from build123d import *

# Parameters (mm, degrees)
SKETCH_1_R          = 60
EXTRUDE_1_DEPTH     = 8
SKETCH_3_R          = 9
EXTRUDE_3_DEPTH     = 36
SKETCH_4_R          = 60
EXTRUDE_4_DEPTH     = 8
SKETCH_5_R          = 15
EXTRUDE_5_DEPTH     = 48
SKETCH_6_R          = 3.3
CUT_EXTRUDE_1_DEPTH = 114.912246927
SKETCH_7_R          = 6
CUT_EXTRUDE_2_DEPTH = 114.912246927
SKETCH_8_R          = 20
CUT_EXTRUDE_3_DEPTH = 8
SKETCH_9_R          = 4.25
CUT_EXTRUDE_4_DEPTH = 20
CHAMFER_1_SIZE      = 1


with BuildPart() as part:
    # 草图1 → 凸台-拉伸1 (new body)
    with BuildSketch(Plane(origin=(0, 40, 0), x_dir=(1, 0, 0), z_dir=(0, 1, 0))):
        with Locations(Location((0, 0, 0), (0, 0, 270))):
            Circle(SKETCH_1_R)
    extrude(amount=EXTRUDE_1_DEPTH)

    # 草图3 → 凸台-拉伸3 (add)
    with BuildSketch(Plane(origin=(0, 40, 0), x_dir=(1, 0, 0), z_dir=(0, 1, 0))):
        with Locations(Location((45, 0, 0), (0, 0, 270))):
            Circle(SKETCH_3_R)
        with Locations(Location((-22.5, -38.971143, 0), (0, 0, 270))):
            Circle(SKETCH_3_R)
        with Locations(Location((-22.5, 38.971143, 0), (0, 0, 270))):
            Circle(SKETCH_3_R)
    extrude(amount=EXTRUDE_3_DEPTH)

    # 草图4 → 凸台-拉伸4 (add)
    with BuildSketch(Plane(origin=(0, 68, 0), x_dir=(1, 0, 0), z_dir=(0, 1, 0))):
        with Locations(Location((0, 0, 0), (0, 0, 270))):
            Circle(SKETCH_4_R)
    extrude(amount=EXTRUDE_4_DEPTH)

    # 草图5 → 凸台-拉伸5 (add)
    with BuildSketch(Plane(origin=(0, 0, 0), x_dir=(1, 0, 0), z_dir=(0, 1, 0))):
        with Locations(Location((0, 0, 0), (0, 0, 270))):
            Circle(SKETCH_5_R)
    extrude(amount=EXTRUDE_5_DEPTH)

    # 草图6 → 切除-拉伸1 (cut, through all)
    with BuildSketch(Plane(origin=(0, 76, 0), x_dir=(1, 0, 0), z_dir=(0, 1, 0))):
        with Locations(Location((45, 0, 0), (0, 0, 270))):
            Circle(SKETCH_6_R)
        with Locations(Location((-22.5, -38.971143, 0), (0, 0, 270))):
            Circle(SKETCH_6_R)
        with Locations(Location((-22.5, 38.971143, 0), (0, 0, 270))):
            Circle(SKETCH_6_R)
    extrude(amount=-CUT_EXTRUDE_1_DEPTH, mode=Mode.SUBTRACT)

    # 草图7 → 切除-拉伸2 (cut, through all)
    with BuildSketch(Plane(origin=(0, 76, 0), x_dir=(1, 0, 0), z_dir=(0, 1, 0))):
        with Locations(Location((22.5, -38.971143, 0), (0, 0, 270))):
            Circle(SKETCH_7_R)
        with Locations(Location((-45, 0, 0), (0, 0, 270))):
            Circle(SKETCH_7_R)
        with Locations(Location((22.5, 38.971143, 0), (0, 0, 270))):
            Circle(SKETCH_7_R)
    extrude(amount=-CUT_EXTRUDE_2_DEPTH, mode=Mode.SUBTRACT)

    # 草图8 → 切除-拉伸3 (cut)
    with BuildSketch(Plane(origin=(0, 76, 0), x_dir=(1, 0, 0), z_dir=(0, 1, 0))):
        with Locations(Location((0, 0, 0), (0, 0, 270))):
            Circle(SKETCH_8_R)
    extrude(amount=-CUT_EXTRUDE_3_DEPTH, mode=Mode.SUBTRACT)

    # 草图9 → 切除-拉伸4 (cut)
    with BuildSketch(Plane(origin=(0, 0, 0), x_dir=(1, 0, 0), z_dir=(0, 1, 0))):
        with Locations(Location((0, 0, 0), (0, 0, 270))):
            Circle(SKETCH_9_R)
    extrude(amount=CUT_EXTRUDE_4_DEPTH, mode=Mode.SUBTRACT)

    # 倒角1
    chamfer_1_edges = [part.edges().sort_by_distance(p)[0] for p in [
        (0, 40, -60),
        (0, 68, -60),
        (0, 76, -60),
        (0, 48, -60),
    ]]
    chamfer(chamfer_1_edges, length=CHAMFER_1_SIZE)


solid = part.part
For this review, take the finished solid that the model builds, in its own axes (mm). A direction names the side the tool comes from. Coordinates: 2 decimals unless noted, no trailing zeros. Loops run counter-clockwise (first coordinate to the right, second up) from the corner with the lowest first, then second, coordinate; pieces in that order, holes last. Notation, with made-up numbers: (-17.75, -20) - (13.25, -20) arc R9 cw to (13.25, -11) - close; hole circle Ø5 at (-39.5, -7). An arc over 180 degrees is marked (long way). Use a Markdown table: item, result. Add a question column.
Item 1: Mouldability with a two-part tool opening along Y and no side actions: class faces 5 (the face through (2.64, 71.96, -59.94)), 6 (the face through (-19.797, 57.86, -30.387)), 7 (the face through (-3.12, 0, 3.12)), 8 (the face through (1, 76, 25)) as pulls with the +Y half, pulls with the -Y half, needs draft (parallel to the pull), parting line crosses it, or undercut.
Item 2: We need section C-C (z = 0). Give the number of separate pieces and of enclosed holes in the cut face, and give its area (3 significant figures).
Item 3: Insertion check: pin 1 Ø7.5 at (x, z) = (-22.5, -38.97) entering from -Y; pin 2 Ø1 at (y, z) = (21.5, -10.5) entering from +X; pin 3 Ø15.5 at (x, z) = (22.5, -38.97) entering from +Y; pin 4 Ø11 at (x, z) = (-45, 0) entering from -Y. Each pin has a flat end and moves straight along its axis. Give the tip position at first contact, or say it passes through.
Item 4: We need section A-A (x = 0). Give the boundary of the cut face in (y, z), and give its area (3 significant figures).
Item 5: We need section D-D (y = 16). Give the boundary of the cut face in (x, z).
Item 6: We need section B-B (y = 71.5). Give the boundary of the cut face in (x, z), and give its area (3 significant figures).
Item 7: Tool access review of faces 1 (the face through (-19.524, 72.056, -4.336)), 2 (the face through (53.923, 57.86, -1.172)), 3 (the face through (2.64, 43.96, -59.94)), 4 (the face through (-12, 40, 12)): name each direction out of +Z, -Z, +X, -X, +Y, -Y from which nothing blocks a thin tool from reaching the whole face with its end or side.
Item 8: For line 1 (X direction, y = 73, z = 0); line 2 (Y direction, x = 4.5, z = 44.5); line 3 (Y direction, x = 32, z = 50.5), list the stretches that pass through material, from the lowest coordinate up.
Results list:
| question | item | result |
|---|---|---|
| 1 | face 5 | needs draft |
| 1 | face 6 | undercut |
| 1 | face 7 | pulls with the -Y half |
| 1 | face 8 | pulls with the +Y half |
| 2 | separate pieces | 5 |
| 2 | enclosed holes | 0 |
| 2 | area | 2,560 mm^2 |
| 3 | pin 1 | stops at y = 40 |
| 3 | pin 2 | stops at x = 11.18 |
| 3 | pin 3 | stops at y = 76 |
| 3 | pin 4 | passes through |
| 4 | outline | (0, -15) - (40, -15) - (40, -59) - (41, -60) - (47, -60) - (48, -59) - (48, 59) - (47, 60) - (41, 60) - (40, 59) - (40, 15) - (0, 15) - (0, 4.25) - (20, 4.25) - (20, -4.25) - (0, -4.25) - close; (68, -59) - (69, -60) - (75, -60) - (76, -59) - (76, -20) - (68, -20) - close; (68, 20) - (76, 20) - (76, 59) - (75, 60) - (69, 60) - (68, 59) - close |
| 4 | area | 2,630 mm^2 |
| 5 | outline | circle Ø30 at (0, 0); hole circle Ø8.5 at (0, 0) |
| 6 | outline | circle Ø120 at (0, 0); hole circle Ø12 at (-45, 0); hole circle Ø6.6 at (-22.5, -38.97); hole circle Ø6.6 at (-22.5, 38.97); hole circle Ø40 at (0, 0); hole circle Ø12 at (22.5, -38.97); hole circle Ø12 at (22.5, 38.97); hole circle Ø6.6 at (45, 0) |
| 6 | area | 9,610 mm^2 |
| 7 | face 1 | +Y |
| 7 | face 2 | none |
| 7 | face 3 | +Y, -Y |
| 7 | face 4 | -Y |
| 8 | line 1 | x = -60 to -51, -39 to -20, 20 to 41.7, 48.3 to 60 |
| 8 | line 2 | y = 40 to 48, 68 to 76 |
| 8 | line 3 | y = 40.79 to 47.21, 68.79 to 75.21 |
